Solid Edge part; units mm, degrees
sketch "Sketch1" plane through (0, 0, 0) normal (0, 0, 1) x (1, 0, 0)
  line L0 (-119.5405, 79.7564) -> (-47.5405, 79.7564)
  line L1 (-47.5405, 79.7564) -> (-47.5405, 151.7564)
  line L2 (-47.5405, 151.7564) -> (-119.5405, 151.7564)
  line L3 (-119.5405, 151.7564) -> (-119.5405, 79.7564)
  line L4 (-123.5405, 75.7564) -> (-43.5405, 75.7564)
  line L5 (-43.5405, 75.7564) -> (-43.5405, 155.7564)
  line L6 (-43.5405, 155.7564) -> (-123.5405, 155.7564)
  line L7 (-123.5405, 155.7564) -> (-123.5405, 75.7564)
  dimension "D1" = 43.5405
  dimension "D2" = 123.5405
extrude "Protrusion1" add sketch "Sketch1" along normal blind 2190
sketch "Sketch2" plane through (-123.5405, 105.7564, 960) normal (-1, 0, 0) x (0, 0, -1)
  circle A0 centre (940, -10) radius 6.1
  circle A1 centre (-1210, -10) radius 6.1
extrude "Cutout1" cut sketch "Sketch2" against normal through all
sketch "Sketch3" plane through (-68.5405, 155.7564, 960) normal (0, 1, 0) x (0, 0, -1)
  line L0 (-1230, -21) -> (-1229.99, -21)
  line L1 (-1229.99, -21) -> (-1229.99, 51)
  line L2 (-1229.99, 51) -> (-1230, 51)
  line L3 (-1230, 51) -> (-1230, -21)
  dimension "D1" = 1229.99
  dimension "D2" = 1229.99
extrude "Cutout2" cut sketch "Sketch3" against normal blind 5
sketch "Sketch4" plane through (-43.5405, 100.7564, 960) normal (1, 0, 0) x (0, 0, 1)
  line L0 (-920, -55) -> (-960, -15)
  line L1 (-960, -15) -> (-960, -55)
  line L2 (-960, -55) -> (-920, -55)
  dimension "D1" = 960
extrude "Cutout3" cut sketch "Sketch4" against normal through all
sketch "Sketch5" plane through (-83.5405, 75.7564, 1095) normal (0, -1, 0) x (0, 0, 1)
  line L0 (995, 36) -> (1095, 36)
  line L1 (1095, 36) -> (1095, -36)
  line L2 (1095, -36) -> (995, -36)
  line L3 (995, -36) -> (995, 36)
  line L4 (-1095, 36) -> (-695, 36)
  line L5 (-695, 36) -> (-695, -36)
  line L6 (-695, -36) -> (-1095, -36)
  line L7 (-1095, -36) -> (-1095, 36)
  dimension "D1" = 1095
  dimension "D2" = 695
  dimension "D3" = 995
  dimension "D4" = 995
extrude "Cutout4" cut sketch "Sketch5" against normal up to next
sketch "Sketch6" plane through (-83.5405, 155.7564, 1115) normal (0, 1, 0) x (0, 0, -1)
  line L0 (-1074.99, -36) -> (-1074.98, -36)
  line L1 (-1074.98, -36) -> (-1074.98, 36)
  line L2 (-1074.98, 36) -> (-1074.99, 36)
  line L3 (-1074.99, 36) -> (-1074.99, -36)
  dimension "D1" = 1074.99
  dimension "D2" = 1074.98
extrude "Cutout5" cut sketch "Sketch6" against normal up to next
fillet "Round1" radius 5 2 edges at (-119.5405, 77.7564, 2090) (-47.5405, 77.7564, 2090)
properties material "Aluminum, 6061-T6"
The listing builds one solid part. Answer for the finished solid, in the listing's coordinates (mm). A direction names the side the tool comes from. Give positions to 0.01 mm unless a question says otherwise; leave off trailing zeros. Order: outer loops, then holes, each group sorted by start corner. A loop starts at its lowest first (then second) coordinate and runs counter-clockwise, first axis right, second up. Notation, with made-up numbers: (-1, -15.5) - (53, -15.5) arc R16 cw to (53, -7.5) - close; hole circle Ø8 at (67.5, 52). An arc over 180 degrees is marked (long way). One line per item, written item: value. Start each with the question number.
1) Given pin 1 Ø16 at (y, z) = (115.76, 2170) entering from +X; pin 2 Ø3 at (x, y) = (-68, 153.5) entering from +Z; pin 3 Ø4.5 at (x, y) = (-84, 77.5) entering from -Z; pin 4 Ø1.2 at (x, y) = (-72, 77) entering from +Z, each flat-ended and moving along its own axis, determine where each tip first touches the part or whether it passes through.
2) A cutting plane is placed at A-A on y = 93.5. Give the vertices of the cut face in (x, z).
3) A cutting plane is placed at C-C on x = -87.5. Give the vertices of the cut face in (y, z), then the cut area to 3 significant figures.
4) A tool of negligible diameter and unlimited length cuts with its end or side. For faces 1 (the face through (-83, 155.756, 1100)), 2 (the face through (-83, 151.756, 1098)), from which of +Z, -Z, +X, -X, +Y, -Y can it reach the whole face along a straight path? Write none if from no direction.
5) The mould has two halves that part along Y. Classify faces 3 (the face through (-83.354, 152.146, 36.39)), 4 (the face through (-119.54, 115, 1080)), 5 (the face through (-84, 75.756, 1323)): released by +Y, released by -Y, zero draft, split by the parting line, or undercut.
6) A cutting plane is placed at D-D on z = 207. Give the vertices of the cut face in (x, y).
7) A cutting plane is placed at B-B on z = 1737.5. Give the vertices of the cut face in (x, y), then the cut area to 3 significant figures.
8) Find the intervals of material crossed by L1, parallel to X at y = 134, z = 1218; L2, parallel to Y at x = -80, z = 1002.5; L3, parallel to Y at x = -45.85, z = 2170, in increasing order.
Answer sheet:
1. pin 1: stops at x = -43.54
1. pin 2: stops at z = 2189.98
1. pin 3: stops at z = 400
1. pin 4: stops at z = 2090
2. outline: (-123.54, 0) - (-119.54, 0) - (-119.54, 2190) - (-123.54, 2190) - close; (-47.54, 0) - (-43.54, 0) - (-43.54, 2190) - (-47.54, 2190) - close
3. outline: (75.76, 400) - (79.76, 400) - (79.76, 2090) - (75.76, 2090) - close; (151.76, 36) - (155.76, 40) - (155.76, 2189.98) - (151.76, 2189.98) - close
3. area: 15,400 mm2
4. face 1: +Z, -Z, +X, -X, +Y
4. face 2: +Z, -Z
5. face 3: released by +Y
5. face 4: undercut
5. face 5: released by -Y
6. outline: (-123.54, 75.76) - (-119.54, 75.76) - (-119.54, 151.76) - (-47.54, 151.76) - (-47.54, 75.76) - (-43.54, 75.76) - (-43.54, 155.76) - (-123.54, 155.76) - close
7. outline: (-123.54, 75.76) - (-43.54, 75.76) - (-43.54, 155.76) - (-123.54, 155.76) - close; hole (-119.54, 79.76) - (-47.54, 79.76) - (-47.54, 151.76) - (-119.54, 151.76) - close
7. area: 1,220 mm2
8. L1: x = -123.54 to -119.54, -47.54 to -43.54
8. L2: y = 75.76 to 79.76, 151.76 to 155.76
8. L3: y = 75.76 to 109.66, 121.86 to 155.76
